Model file for the job. Use its own axes, mm. Face numbers are marked on the shaded views. A direction names the side the tool comes from. Coordinates: 2 decimals unless noted, no trailing zeros. Loops run counter-clockwise (first coordinate to the right, second up) from the corner with the lowest first, then second, coordinate; pieces in that order, holes last.
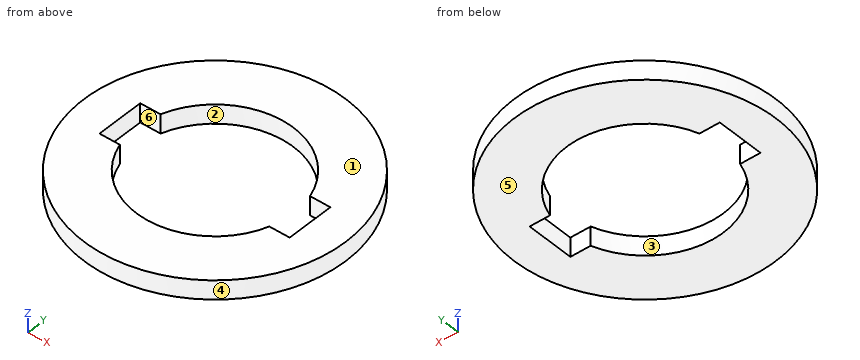
Autodesk Fusion 360 part; units mm, degrees
sketch "Sketch1" plane through (0, 0, 0) normal (0, 0, 1) x (1, 0, 0)
  circle A0 centre (0, 0) radius 27.5
  circle A1 centre (0, 0) radius 16.5
  dimension "d1" = 55
  dimension "d2" = 33
extrude "Extrude1" add sketch "Sketch1" along normal blind 4
sketch "Sketch2" plane through (0, 0, 4) normal (0, 0, 1) x (-1, 0, 0)
  circle A0 centre (0, 0) radius 16.5
  circle A1 centre (0, 0) radius 27.5
  line L0 (20, -5) -> (-20, -5)
  line L1 (-20, -5) -> (-20, 5)
  line L2 (-20, 5) -> (20, 5)
  line L3 (20, 5) -> (20, -5)
extrude "Extrude2" cut sketch "Sketch2" against normal blind 15 contours A0 L0 L2 L3 | A0 L0 L1 L2
Q1. Slice it at A-A (y = 0). List the corners of the cut face in (x, z), and give its area (3 significant figures).
Answers:
outline: (-27.5, 0) - (-20, 0) - (-20, 4) - (-27.5, 4) - close; (20, 0) - (27.5, 0) - (27.5, 4) - (20, 4) - close
area: 60.0 mm2
Q2. Mould opens along X. For the marked faces 3, 4, 5 and 6 say: +X half, -X half, draft (parallel to the pull), parting line (faces both ways), or undercut.
Answers:
face 3: undercut
face 4: parting line
face 5: draft
face 6: undercut
Q3. Slice it at B-B (x = 0). List the corners of the cut face in (y, z).
Answers:
outline: (-27.5, 0) - (-16.5, 0) - (-16.5, 4) - (-27.5, 4) - close; (16.5, 0) - (27.5, 0) - (27.5, 4) - (16.5, 4) - close
Q4. Flat gauge pins, fed straight in: P1, Ø1, axis at y = -14.5, z = 2, coming from the +X side; P2, Ø1.2, axis at x = -18.5, z = 3, coming from the -Y side; P3, Ø2, axis at x = 20, y = -13, coming from the -Z side; P4, Ø1.5, axis at y = 20, z = 3, coming from the -X side. Where does each tip first touch, or does it go through?
Answers:
P1: stops at x = 23.67
P2: stops at y = -20.88
P3: stops at z = 0
P4: stops at x = -19.64
Q5. Slice it at C-C (z = 3.1). List the corners of the cut face in (x, y).
Answers:
outline: circle Ø55 at (0, 0); hole (-20, -5) - (-15.72, -5) arc R16.5 ccw to (15.72, -5) - (20, -5) - (20, 5) - (15.72, 5) arc R16.5 ccw to (-15.72, 5) - (-20, 5) - close
Q6. Which spindle directions (+Z, -Z, +X, -X, +Y, -Y) get a long thin tool onto all of the face, cutting with end or side? Do the marked faces 1 and 2. Say none if no direction does.
Answers:
face 1: +Z, +X, -X, +Y, -Y
face 2: +Z, -Z
Q7. Slice it at D-D (y = 18.5). List the corners of the cut face in (x, z), and give its area (3 significant figures).
Answers:
outline: (-20.35, 0) - (20.35, 0) - (20.35, 4) - (-20.35, 4) - close
area: 163 mm2
Q8. Drill centre lines: line 1 (Y direction, x = -0.5, z = 2.4); line 2 (X direction, y = 0.5, z = 0.9); line 3 (X direction, y = -14, z = 3.65). Where is each one in solid material? Low to high.
Answers:
line 1: y = -27.5 to -16.49, 16.49 to 27.5
line 2: x = -27.5 to -20, 20 to 27.5
line 3: x = -23.67 to -8.73, 8.73 to 23.67
